from build123d import *

# Parameters (mm, degrees)
SKETCH1_R           = 5
BOSS_EXTRUDE2_DEPTH = 10


with BuildPart() as part:
    # Sketch1 → Boss-Extrude2 (new body)
    with BuildSketch(Plane.XY):
        Polygon((25, 12.144578313), (-25, 12.144578313), (-35, 2.144578313), (-35, -37.855421687), (-25, -37.855421687), (-25, -27.855421687), (-15, -27.855421687), (-15, -37.855421687), (15, -37.855421687), (15, -27.855421687), (25, -27.855421687), (25, -37.855421687), (35, -37.855421687), (35, 2.144578313), align=None)
        with Locations((-25, 2.144578313)):
            Circle(SKETCH1_R, mode=Mode.SUBTRACT)
        with Locations(Location((25, 2.144578313, 0), (0, 0, 180))):
            Circle(SKETCH1_R, mode=Mode.SUBTRACT)
        Polygon((5.421686747, -17.855421687), (-5.421686747, -17.855421687), (-5.421686747, -12.855421687), (-15.421686747, -12.855421687), (-15.421686747, -22.855421687), (15.421686747, -22.855421687), (15.421686747, -12.855421687), (5.421686747, -12.855421687), align=None, mode=Mode.SUBTRACT)
    extrude(amount=BOSS_EXTRUDE2_DEPTH)


solid = part.part
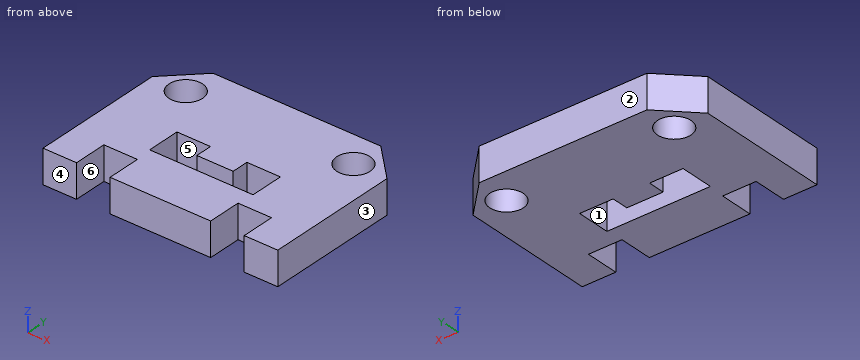
Here's how the part is built. I have some questions about the finished solid (model axes, mm). Face numbers are marked on the shaded views. A direction names the side the tool comes from. Round coordinates to 2 decimals unless told otherwise and drop trailing zeros. Loops run counter-clockwise (first coordinate to the right, second up) from the corner with the lowest first, then second, coordinate; pieces in that order, holes last.
1. Which directions (+Z, -Z, +X, -X, +Y, -Y) give clear straight access to the entire face, cutting with the end or side of a thin tool? Please do the marked faces 4, 5 and 6.
Answer list:
face 4: +Z, -Z, +X, -X, -Y
face 5: +Z, -Z
face 6: +Z, -Z, -Y
2. If we section it at C-C on y = 3.5: Write out the boundary of the cut face in (x, z).
Answer list:
outline: (-33.64, 0) - (-29.81, 0) - (-29.81, 10) - (-33.64, 10) - close; (-20.19, 0) - (20.19, 0) - (20.19, 10) - (-20.19, 10) - close; (29.81, 0) - (33.64, 0) - (33.64, 10) - (29.81, 10) - close
3. If we section it at D-D on x = 22.5: Write out the boundary of the cut face in (y, z).
Answer list:
outline: (-27.86, 0) - (-2.19, 0) - (-2.19, 10) - (-27.86, 10) - close; (6.47, 0) - (12.14, 0) - (12.14, 10) - (6.47, 10) - close
4. If I drill on line 1 along X through (y, z) = (-17, 4.25); line 2 along X through (y, z) = (-31, 5.25); line 3 along Y through (x, z) = (-9, 8.5), over which ranges is the centre line in solid material (lowest first)?
Answer list:
line 1: x = -35 to -15.42, -5.42 to 5.42, 15.42 to 35
line 2: x = -35 to -25, -15 to 15, 25 to 35
line 3: y = -37.86 to -22.86, -12.86 to 12.14
5. If we section it at A-A on x = -7: Write out the boundary of the cut face in (y, z).
Answer list:
outline: (-37.86, 0) - (-22.86, 0) - (-22.86, 10) - (-37.86, 10) - close; (-12.86, 0) - (12.14, 0) - (12.14, 10) - (-12.86, 10) - close
6. We'd pull the mould along X, two halves only. Please class the marked faces 1, 2 and 3: +X half, -X half, draft (parallel to the pull), parting line (faces both ways), or undercut.
Answer list:
face 1: undercut
face 2: draft
face 3: +X half
7. If we section it at B-B on z = 2.75: Write out the boundary of the cut face in (x, y), plus the area to 3 significant figures.
Answer list:
outline: (-35, -37.86) - (-25, -37.86) - (-25, -27.86) - (-15, -27.86) - (-15, -37.86) - (15, -37.86) - (15, -27.86) - (25, -27.86) - (25, -37.86) - (35, -37.86) - (35, 2.14) - (25, 12.14) - (-25, 12.14) - (-35, 2.14) - close; hole circle Ø10 at (-25, 2.14); hole (-15.42, -22.86) - (15.42, -22.86) - (15.42, -12.86) - (5.42, -12.86) - (5.42, -17.86) - (-5.42, -17.86) - (-5.42, -12.86) - (-15.42, -12.86) - close; hole circle Ø10 at (25, 2.14)
area: 2,790 mm2
8. For P1, Ø4, axis at x = 3.5, y = -3.5, coming from the -Z side; P2, Ø3, axis at x = 18, z = 5, coming from the -Y side, each with a flat end and sliding along its axis, tell me the tip position at first contact or that it passes through.
Answer list:
P1: stops at z = 0
P2: stops at y = -27.86
